Part model, mm, in its own coordinate system. Face numbers are marked on the shaded views. A direction names the side the tool comes from. Round coordinates to 2 decimals unless told otherwise and drop trailing zeros. Write each loop counter-clockwise with the first axis right and the second up, starting at its lowest first coordinate (ties: lowest second). Pieces come first, ordered by that corner, then holes. Notation, with made-up numbers: M 20.25,-14.75 L 60.25,-14.75 A16 ccw 60.25,11.25 Z; hole C 20.25,75 d7. An arc over 180 degrees is marked long. One line per question, with ' | ' between items. Start each with the question number.
1) Wall check: probe 1 along X at (y, z) = (-10.5, 4); probe 2 along Y at (x, z) = (11, 17); probe 3 along X at (y, z) = (-9, 16). Give the ranges that are in metal, low to high. Write a range as [from, to].
2) Saw through at D-D (z = 9). List the corners of the cut face in (x, y).
3) Saw through at B-B (z = 25.5). List the corners of the cut face in (x, y), plus the area to 3 significant figures.
4) Drop flat-ended pins along their axis: pin 1 Ø17.5 at (x, y) = (-24.5, 0) entering from -Z; pin 2 Ø1.5 at (y, z) = (-11, 19.5) entering from -X; pin 3 Ø1.1 at (x, z) = (12, 0.5) entering from -Y; pin 4 Ø0.6 at (y, z) = (-3, -1) entering from +X. Give the stop position or say it passes through.
5) Tool access for the marked faces 1, 2, 3 and 4: list every direction of +Z, -Z, +X, -X, +Y, -Y with a clear straight run to the whole face (end or side of a thin tool).
6) Saw through at A-A (x = -65). List the corners of the cut face in (y, z), plus the area to 3 significant figures.
7) Mould opens along Y. For the marked faces 5, 6 and 7 say: pulls with the +Y half, pulls with the -Y half, needs draft (parallel to the pull), parting line crosses it, or undercut.
8) Saw through at C-C (y = 0). Give the number of separate pieces and of enclosed holes in the cut face, plus the area to 3 significant figures.
```python
from build123d import *

# Parameters (mm, degrees)
F0_W     = 84
F0_H     = 36
F0_W_2   = 80
F0_H_2   = 32
F1_DEPTH = 30
F0_W_3   = 76
F0_H_3   = 28
F2_DEPTH = 3
F0_R     = 11
F3_DEPTH = 2
F4_SIZE  = 1.99999
F5_SIZE  = 1.99999
F6_W     = 27
F6_H     = 1.99999
F7_DEPTH = 5
F9_DEPTH = 15.3
F10_R    = 0.99999


# Not quite as in the source:
# - a fillet or chamfer is up to 0.001 mm smaller than in the source, because OpenCascade refuses the exact size


with BuildPart() as f1:
    # F0 (on Top) → F1 (new body)
    with BuildSketch(Plane.XY):
        Rectangle(F0_W, F0_H)
        Rectangle(F0_W_2, F0_H_2, mode=Mode.SUBTRACT)
    extrude(amount=F1_DEPTH)

    # F0 (on Top) → F2 (join)
    with BuildSketch(Plane.XY):
        Rectangle(F0_W_2, F0_H_2)
        Rectangle(F0_W_3, F0_H_3, mode=Mode.SUBTRACT)
    extrude(amount=F2_DEPTH)

    # F0 (on Top) → F3 (join)
    with BuildSketch(Plane.XY):
        Rectangle(F0_W_2, F0_H_2)
        Rectangle(F0_W_3, F0_H_3, mode=Mode.SUBTRACT)
        Rectangle(F0_W_3, F0_H_3)
        with Locations((-24.4961753488, 0)):
            Circle(F0_R, mode=Mode.SUBTRACT)
    extrude(amount=-F3_DEPTH)

    # F4 (size 2 in the source; OpenCascade refuses exactly that, so slightly less here)
    f4_edges = [f1.edges().sort_by_distance(p)[0] for p in [
        (0, 18, 0),
        (0, -18, 0),
        (42, 0, 0),
        (-42, 0, 0),
    ]]
    chamfer(f4_edges, length=F4_SIZE)

    # F5 (size 2 in the source; OpenCascade refuses exactly that, so slightly less here)
    f5_edges = [f1.edges().sort_by_distance(p)[0] for p in [
        (0, -14, 3),
        (38, 0, 3),
        (0, 14, 3),
        (-38, 0, 3),
    ]]
    chamfer(f5_edges, length=F5_SIZE)

    # F6 (on face) → F7 (cut)
    with BuildSketch(Plane(origin=(-42, 0, 0), x_dir=(0, -1, 0), z_dir=(-1, 0, 0))):
        with Locations((0, 0.999995)):
            Rectangle(F6_W, F6_H)
    extrude(amount=-F7_DEPTH, mode=Mode.SUBTRACT)

    # F8 (on face) → F9 (join)
    with BuildSketch(Plane(origin=(0, 0, -2), x_dir=(1, 0, 0), z_dir=(0, 0, -1))):
        Polygon((-40, 14), (-40, 16), (-75, 16), (-75, -16), (-40, -16), (-40, -14), (-73, -14), (-73, 14), align=None)
    extrude(amount=-F9_DEPTH)

    # F10 (radius 1 in the source; OpenCascade refuses exactly that, so slightly less here)
    f10_edges = [f1.edges().sort_by_distance(p)[0] for p in [
        (-35.496175, 0, -2),
        (-35.496175, 0, 0),
    ]]
    fillet(f10_edges, radius=F10_R)


solid = f1.part
```
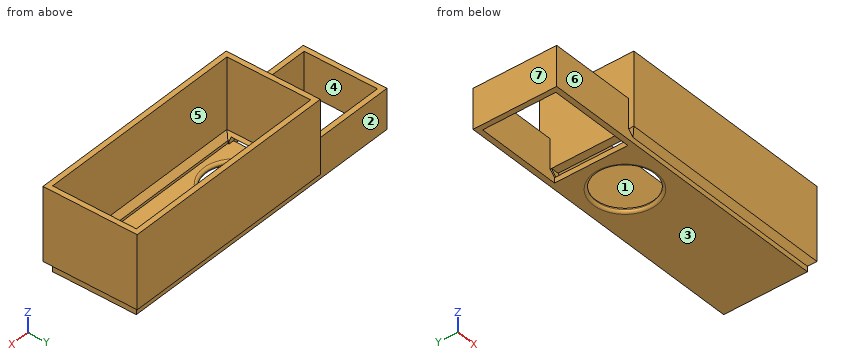
Answer key:
1) probe 1: x = [-75, -73], [-42, -40], [40, 42] | probe 2: y = [-18, -16], [16, 18] | probe 3: x = [-42, -40], [40, 42]
2) outline: M -75,-16 L -42,-16 L -42,-18 L 42,-18 L 42,18 L -42,18 L -42,16 L -75,16 Z; hole M -73,-14 L -42,-14 L -42,14 L -73,14 Z; hole M -40,-16 L 40,-16 L 40,16 L -40,16 Z
3) outline: M -42,-18 L 42,-18 L 42,18 L -42,18 Z; hole M -40,-16 L 40,-16 L 40,16 L -40,16 Z | area: 464 mm2
4) pin 1: passes through | pin 2: stops at x = -42 | pin 3: stops at y = -17.05 | pin 4: stops at x = 40
5) face 1: +Z | face 2: -Z, -X, +Y | face 3: -Z, +X, -X, +Y, -Y | face 4: +Z, -Z
6) outline: M -16,-2 L -14,-2 L -14,13.3 L -16,13.3 Z; M 14,-2 L 16,-2 L 16,13.3 L 14,13.3 Z | area: 61.2 mm2
7) face 5: undercut | face 6: pulls with the -Y half | face 7: needs draft
8) separate pieces: 4 | enclosed holes: 0 | area: 264 mm2
